from build123d import *

# Parameters (mm, degrees)
SKETCH1_W           = 90
SKETCH1_H           = 41.35
BOSS_EXTRUDE1_DEPTH = 3.175
SKETCH3_W           = 6.35
SKETCH3_H           = 13.175
LEFTRIGHT_DEPTH     = 50.927729019
SKETCH4_W           = 14.5
SKETCH4_H           = 16.1
RIGHT_DEPTH         = 50.927729019


with BuildPart() as part:
    # Sketch1 → Boss-Extrude1 (new, symmetric)
    with BuildSketch(Plane(origin=(0, 0, 0), x_dir=(1, 0, 0), z_dir=(0, 1, 0))):
        Rectangle(SKETCH1_W, SKETCH1_H)
    extrude(amount=BOSS_EXTRUDE1_DEPTH, both=True)

    # Sketch3 → LeftRight (cut, through all)
    with BuildSketch(Plane(origin=(0, 3.175, 0), x_dir=(1, 0, 0), z_dir=(0, 1, 0))):
        with Locations((-41.825, -14.0875)):
            Rectangle(SKETCH3_W, SKETCH3_H)
        with Locations((-41.825, 14.0875)):
            Rectangle(SKETCH3_W, SKETCH3_H)
        with Locations((41.825, 14.0875)):
            Rectangle(SKETCH3_W, SKETCH3_H)
        with Locations((41.825, -14.0875)):
            Rectangle(SKETCH3_W, SKETCH3_H)
    extrude(amount=-LEFTRIGHT_DEPTH, mode=Mode.SUBTRACT)

    # Sketch4 → Right (cut, through all)
    with BuildSketch(Plane.XZ.offset(3.175)):
        with Locations((-17.74, -3.742440275)):
            Rectangle(SKETCH4_W, SKETCH4_H)
    extrude(amount=-RIGHT_DEPTH, mode=Mode.SUBTRACT)


solid = part.part
The listing builds one solid part. Answer for the finished solid, in the listing's coordinates (mm). A direction names the side the tool comes from. Give positions to 0.01 mm unless a question says otherwise; leave off trailing zeros. Write each loop counter-clockwise with the first axis right and the second up, starting at its lowest first coordinate (ties: lowest second). Pieces come first, ordered by that corner, then holes.
1) For a pull along Z with two mould halves and no side action, classify faces 1 (the face through (-18, 0, 4.308)), 2 (the face through (-18, 0, -11.792)), 3 (the face through (-45, 0, 0)), 4 (the face through (-1, 0, -20.675)) as pulls with the +Z half, pulls with the -Z half, needs draft (parallel to the pull), parting line crosses it, or undercut.
2) Section A-A (z = 0) is taken. Write down the section's boundary in (x, y) (3 decimals), and give its area (3 significant figures).
3) Find the intervals of material crossed by L1, parallel to X at y = 0.25, z = -4; L2, parallel to X at y = 1.5, z = -10; L3, parallel to X at y = 1.5, z = 16, in increasing order.
4) Section B-B (y = -0.25) is taken. Write down the section's boundary in (x, z) (3 decimals), and give its area (3 significant figures).
5) A tool of negligible diameter and unlimited length cuts with its end or side. For faces 5 (the face through (-10.49, 0, -4)), 6 (the face through (-42, 0, -7.5)), 7 (the face through (42, 0, 7.5)), 8 (the face through (-38.65, 0, 14)), from which of +Z, -Z, +X, -X, +Y, -Y can it reach the whole face along a straight path? Write none if from no direction.
6) Section C-C (x = -17.5) is taken. Write down the section's boundary in (y, z) (3 decimals).
7) Given P1, Ø3, axis at y = 0.5, z = -15, coming from the -X side; P2, Ø2, axis at y = -0.5, z = -13.5, coming from the +X side, each flat-ended and moving along its own axis, determine where each tip first touches the part or whether it passes through.
8) Section D-D (z = -15) is taken. Write down the section's boundary in (x, y) (3 decimals).
Response:
1. face 1: undercut
1. face 2: undercut
1. face 3: needs draft
1. face 4: pulls with the -Z half
2. outline: (-45, -3.175) - (-24.99, -3.175) - (-24.99, 3.175) - (-45, 3.175) - close; (-10.49, -3.175) - (45, -3.175) - (45, 3.175) - (-10.49, 3.175) - close
2. area: 479 mm2
3. L1: x = -45 to -24.99, -10.49 to 45
3. L2: x = -38.65 to -24.99, -10.49 to 38.65
3. L3: x = -38.65 to 38.65
4. outline: (-45, -7.5) - (-38.65, -7.5) - (-38.65, -20.675) - (38.65, -20.675) - (38.65, -7.5) - (45, -7.5) - (45, 7.5) - (38.65, 7.5) - (38.65, 20.675) - (-38.65, 20.675) - (-38.65, 7.5) - (-45, 7.5) - close; hole (-24.99, -11.792) - (-10.49, -11.792) - (-10.49, 4.308) - (-24.99, 4.308) - close
4. area: 3,150 mm2
5. face 5: +Y, -Y
5. face 6: -Z, -X, +Y, -Y
5. face 7: +Z, +X, +Y, -Y
5. face 8: +Z, -X, +Y, -Y
6. outline: (-3.175, -20.675) - (3.175, -20.675) - (3.175, -11.792) - (-3.175, -11.792) - close; (-3.175, 4.308) - (3.175, 4.308) - (3.175, 20.675) - (-3.175, 20.675) - close
7. P1: stops at x = -38.65
7. P2: stops at x = 38.65
8. outline: (-38.65, -3.175) - (38.65, -3.175) - (38.65, 3.175) - (-38.65, 3.175) - close
